Autodesk Inventor part; units mm, degrees
ref_plane "YZ Plane" through (0, 0, 0) normal (1, 0, 0) x (0, 1, 0)
ref_plane "XZ Plane" through (0, 0, 0) normal (0, 1, 0) x (-1, 0, 0)
ref_plane "XY Plane" through (0, 0, 0) normal (0, 0, 1) x (1, 0, 0)
sketch "Sketch1" plane through (0, 0, 0) normal (0, 0, 1) x (1, 0, 0)
  circle A0 centre (0, 0) radius 5.461
  dimension "d0" = 10.922
extrude "Extrusion1" add sketch "Sketch1" along normal blind 6.096
sketch "Sketch2" plane through (0, 0, 0) normal (0, 0, -1) x (-1, 0, 0)
  circle A0 centre (0, 0) radius 5.461
  line L0 (0, -35) -> (0, 35)
  line L1 (35, 0) -> (-35, 0)
  line L2 (0, 1.4986) -> (25, 1.4986)
  line L3 (25, 1.4986) -> (25, -1.4986)
  line L4 (25, -1.4986) -> (0, -1.4986)
  line L5 (0, -1.4986) -> (0, 1.4986)
  line L6 (-1.2978, -0.7493) -> (-13.7978, 20.9013)
  line L7 (-13.7978, 20.9013) -> (-11.2022, 22.3999)
  line L8 (-11.2022, 22.3999) -> (1.2978, 0.7493)
  line L9 (1.2978, 0.7493) -> (-1.2978, -0.7493)
  line L10 (1.2978, -0.7493) -> (-11.2022, -22.3999)
  line L11 (-11.2022, -22.3999) -> (-13.7978, -20.9013)
  line L12 (-13.7978, -20.9013) -> (-1.2978, 0.7493)
  line L13 (-1.2978, 0.7493) -> (1.2978, -0.7493)
  circle A1 centre (0, 0) radius 25
  point P0 (25, 0)
  point P1 (-12.5, 21.6506)
  point P2 (-12.5, -21.6506)
  dimension "d3" = 2.9972
  dimension "d6" = 360
  dimension "d8" = 50
extrude "Extrusion2" add sketch "Sketch2" against normal blind 4 contours L1 L9 L8 L2 A0 | L1 A1 L4 A0 | A0 L2 A1 L1 | A0 L4 L10 L13 L1 | A1 L2 L3 | L3 L4 A1 | L13 L10 L4 L0 | L13 L12 L6 A0 L8 L0 | L9 L6 L1 | L0 L2 L8 L9 | L0 L10 A0 L12 L6 L9 | L1 L12 L13 | L2 L0 L8 | L10 L0 L4 | A0 L6 A1 L8 | L10 A1 L12 A0 | A1 L7 L8 | L10 L11 A1 | L6 L7 A1 | A1 L11 L12
sketch "Sketch6" plane through (0, 0, 0) normal (0, 0, -1) x (-1, 0, 0)
  line L0 (5.2514, 1.4986) -> (25, 1.4986)
  arc A0 (-3.9235, 3.7985) -> (-3.9235, -3.7985) centre (0, 0) ccw
  circle A1 centre (0, 0) radius 23.094
  line L1 (0, 0) -> (27, 0)
  line L2 (0, 0) -> (-13.5, -23.3827)
  line L3 (0, 0) -> (-13.5, 23.3827)
  point P0 (-11.547, 20)
  point P1 (23.094, 0)
  dimension "d26" = 360
  dimension "d28" = 40
hole "Hole2" at (-23.094, 0, 0) direction (0, 0, 1) diameter 0.515 end through all
pattern_circular "Circular Pattern2" count 3 over 360 about axis through (0, 0, -10) along (0, 0, 1) of "Hole2"
sketch "Sketch8" plane through (11.2022, -22.3999, 0) normal (0.5, -0.8660254, 0) x (0.8660254, 0.5, 0)
  line L0 (2.9972, 4) -> (0, 4)
  line L1 (1.4986, -1.2192) -> (1.4986, 7.3152)
  line L2 (1.4986, 4) -> (1.4986, 0)
  point P0 (1.4986, 2)
hole "Hole4" at (12.5, -21.6506, 2) direction (-0.5, 0.8660254, 0) diameter 1.181 depth 1.906
pattern_circular "Circular Pattern3(Side_hole)" count 3 over 360 about axis through (0, 0, -10) along (0, 0, 1) of "Hole4"
sketch "Sketch18" plane through (0, 0, 6.096) normal (0, 0, 1) x (1, 0, 0)
  circle A0 centre (0, 0) radius 5.461
  line L0 (-32.72, 0) -> (21.3198, 0)
  point P0 (3.81, 0)
  point P1 (-1.905, 3.2996)
  point P2 (-1.905, -3.2996)
  dimension "d87" = 3.81
  dimension "d90" = 360
hole "Hole7" at (-1.905, 3.2996, 6.096) at (-1.905, -3.2996, 6.096) direction (0, 0, -1) diameter 1.4732 end through all
sketch "Sketch22" plane through (0, 0, 0) normal (0, 0, -1) x (-1, 0, 0)
  arc A0 (-1.3279, -5.2971) -> (5.2514, -1.4986) centre (0, 0) ccw
  circle A1 centre (0, 0) radius 1.4986
  dimension "d104" = 2.9972
extrude "Extrusion9" add sketch "Sketch22" along normal blind 5.08
sketch "Sketch23" plane through (0, 0, 6.096) normal (0, 0, 1) x (1, 0, 0)
  circle A0 centre (0, 0) radius 5.461
hole "Hole8" at (0, 0, 6.096) direction (0, 0, -1) diameter 1.778 end through all
properties part number "TriPost" material "Aluminum-6061"
Input: part model. Units: mm. Frame: model coordinates. A direction names the side the tool comes from. Coordinates: 2 decimals unless noted, no trailing zeros. Order: outer loops, then holes, each group sorted by start corner. A loop starts at its lowest first (then second) coordinate and runs counter-clockwise, first axis right, second up. Notation, with made-up numbers: M -33.5,78 L -25.5,78 A14 cw -25.5,90 Z; hole C -10.75,2 d8. An arc over 180 degrees is marked long. Write item = value, one per line. Start each with the question number.
(1) Reachability of faces 1 (the flat face through (-15, -1.499, 2)), 2 (the flat face through (13.059, -21.328, 2.416)), 3 (the cylindrical face through (-1.62, -3.98, 3.01)), 4 (the flat face through (8.93, -12.47, 1.97)), 5 (the cylindrical face through (5.21, -1.64, 3.01)) from +Z, -Z, +X, -X, +Y, -Y: full face, straight path, thin tool, end or side. Return the list, or none.
(2) First-contact query: P1, Ø13.5, axis at x = 8, y = -10.5, coming from the +Z side; P2, Ø1.2, axis at x = -10.5, z = 2, coming from the -Y side; P3, Ø6, axis at x = 3.5, z = 2.5, coming from the -Y side. Flat tips, straight axial feed; report the tip coordinate or a pass-through.
(3) Section D-D on x = -17.5. Output: boundary loops of the cut face in (y, z).
(4) Section A-A on x = 0. Output: boundary loops of the cut face in (y, z), and give its area (3 significant figures).
(5) Section C-C on z = 2. Give the number of separate pieces and of enclosed holes in the cut face, and give its area (3 significant figures).
(6) Line query: line 1 along Y through (x, z) = (-23.8, 2); line 2 along Y through (x, z) = (4.5, 2); line 3 along Y through (x, z) = (4, 1.5). Output: solid intervals per line, ascending. Write a range as [from, to].
(7) Pull-direction query (X, two-part tool) for faces 6 (the cylindrical face through (11.99, -20.83, 2.59)), 7 (the flat face through (11.941, 21.973, 2.416)), 8 (the flat face through (1.1, 0.1, 6.096)), 9 (the cylindrical face through (-1.43, -0.45, -2.5)); classes: released by +X, released by -X, zero draft, split by the parting line, or undercut.
(8) Section B-B on z = -4. Output: boundary loops of the cut face in (x, y), and give its area (3 significant figures).
Result set:
q1.face_1 = +Z, -Z, -X, -Y
q1.face_2 = +Z, -Z, +X, -Y
q1.face_3 = +Z, -Z
q1.face_4 = +Z, -Z, +X
q1.face_5 = +Z
q2.P1 = 4
q2.P2 = -1.5
q2.P3 = -14.26
q3.outline = M -1.5,0 L 1.5,0 L 1.5,4 L -1.5,4 Z
q4.outline = M -5.46,0 L -1.5,0 L -1.5,-5.08 L -0.89,-5.08 L -0.89,6.1 L -5.46,6.1 Z; M 0.89,-5.08 L 1.5,-5.08 L 1.5,0 L 5.46,0 L 5.46,6.1 L 0.89,6.1 Z
q4.area = 61.9 mm²
q5.separate_pieces = 1
q5.enclosed_holes = 3
q5.area = 257 mm²
q6.line_1 = [-1.5, -0.59], [0.59, 1.5]
q6.line_2 = [-10.79, -4.8], [-3.09, 3.09], [4.8, 10.79]
q6.line_3 = [-9.93, -3.93], [-3.72, 3.72], [3.93, 9.93]
q7.face_6 = undercut
q7.face_7 = released by +X
q7.face_8 = zero draft
q7.face_9 = split by the parting line
q8.outline = C 0,0 d3; hole C 0,0 d1.78
q8.area = 4.57 mm²
